Verification items for this drawing (mm, ordinates from the low corner). A direction names the side the tool comes from. Give positions to 0.01 mm unless a question says otherwise; leave off trailing zeros. Write each loop counter-clockwise with the first axis right and the second up, starting at its lowest first coordinate (ties: lowest second). Pieces come first, ordered by that corner, then holes. Notation, with made-up numbers: (-34.75, -35.75) -> (23.25, -35.75) arc R22 ccw to (23.25, -16.75) -> close; hole circle Ø8 at (48, 89.25). An arc over 180 degrees is marked (long way). Write item = value, one per line.
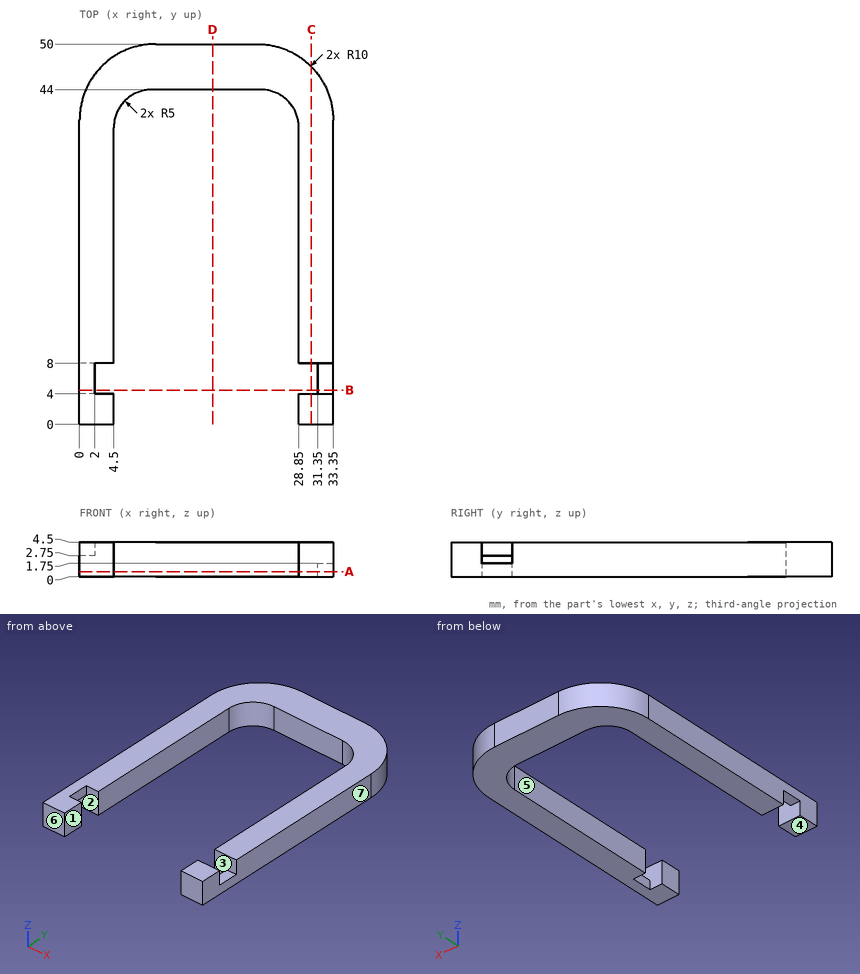
Item 1: Sectioned sample at C-C on x = 30.5. Record the cut outline in (y, z).
Response values:
outline = (0, 0) -> (4, 0) -> (4, 4.5) -> (0, 4.5) -> close; (8, 0) -> (46.99, 0) -> (46.99, 4.5) -> (8, 4.5) -> close
Item 2: Sectioned sample at B-B on y = 4.5. Record the cut outline in (x, z), then the cut area to 3 significant figures.
Response values:
outline = (0, 2.75) -> (2, 2.75) -> (2, 4.5) -> (0, 4.5) -> close; (31.35, 0) -> (33.35, 0) -> (33.35, 1.75) -> (31.35, 1.75) -> close
area = 7.00 mm^2
Item 3: Material ranges on line 1 (X direction, y = 23.5, z = 1.7); line 2 (Y direction, x = 20, z = 3.45); line 3 (Y direction, x = 4, z = 3.5), recorded low to high.
Response values:
line_1 = 0 to 4.5, 28.85 to 33.35
line_2 = 44 to 50
line_3 = 0 to 4, 8 to 48
Item 4: Sectioned sample at A-A on z = 0.65. Record the cut outline in (x, y).
Response values:
outline = (0, 0) -> (4.5, 0) -> (4.5, 4) -> (0, 4) -> close; (0, 8) -> (4.5, 8) -> (4.5, 39) arc R5 cw to (9.5, 44) -> (23.85, 44) arc R5 cw to (28.85, 39) -> (28.85, 8) -> (31.35, 8) -> (31.35, 4) -> (28.85, 4) -> (28.85, 0) -> (33.35, 0) -> (33.35, 40) arc R10 ccw to (23.35, 50) -> (10, 50) arc R10 ccw to (0, 40) -> close
Item 5: Sectioned sample at D-D on x = 17.5. Record the cut outline in (y, z).
Response values:
outline = (44, 0) -> (50, 0) -> (50, 4.5) -> (44, 4.5) -> close
Item 6: Go/stop test with flat-tipped pins: P1, Ø2, axis at x = 32, z = 1.5, coming from the +Y side; P2, Ø1.9, axis at y = 6, z = 0.5, coming from the -X side; P3, Ø2, axis at x = 15, z = 3, coming from the -Y side; P4, Ø1.5, axis at x = 22, y = 42.5, coming from the +Z side. Record where each tip stops, or that it passes through.
Response values:
P1 = 46.44
P2 = 31.35
P3 = 44
P4 = through
Item 7: Set-up check for the marked faces 1, 2, 3 and 4: record each of +Z, -Z, +X, -X, +Y, -Y from which the full face is reachable in a straight line by a thin tool's end or side.
Response values:
face_1 = +Z, -Z, -Y
face_2 = -Z
face_3 = +Z
face_4 = -Z, +X, -X, +Y, -Y
Item 8: Mould release check, pull along X, two halves, no side actions. Record for the marked faces 5, 6 and 7: +X half, -X half, draft (parallel to the pull), parting line (faces both ways), or undercut.
Response values:
face_5 = undercut
face_6 = draft
face_7 = +X half
